```python
from build123d import *

# Parameters (mm, degrees)
SKETCH_1_W          = 200
SKETCH_1_H          = 180
EXTRUDE_1_DEPTH     = 3
SKETCH_2_R          = 1.5
CUT_EXTRUDE_1_DEPTH = 3
SKETCH_3_R          = 1.5
CUT_EXTRUDE_2_DEPTH = 3
SKETCH_4_R          = 2.137012609
SKETCH_4_R_2        = 2.00688496
SKETCH_4_R_3        = 1.920113274
CUT_EXTRUDE_3_DEPTH = 3


with BuildPart() as part:
    # 草图1 → 凸台-拉伸1 (new body)
    with BuildSketch(Plane(origin=(0, 0, 0), x_dir=(1, 0, 0), z_dir=(0, 1, 0))):
        Rectangle(SKETCH_1_W, SKETCH_1_H)
    extrude(amount=EXTRUDE_1_DEPTH)

    # 草图2 → 切除-拉伸1 (cut)
    with BuildSketch(Plane(origin=(0, 3, 0), x_dir=(1, 0, 0), z_dir=(0, 1, 0))):
        with Locations(Location((91.756220162, 76.163438047, 0), (0, 0, 270))):
            Circle(SKETCH_2_R)
        with Locations(Location((91.756220162, 11.939610887, 0), (0, 0, 270))):
            Circle(SKETCH_2_R)
        with Locations(Location((91.756220162, -50.625190386, 0), (0, 0, 270))):
            Circle(SKETCH_2_R)
        with Locations(Location((-91.756220162, 76.163438047, 0), (0, 0, 90))):
            Circle(SKETCH_2_R)
        with Locations(Location((-91.756220162, 11.939610887, 0), (0, 0, 90))):
            Circle(SKETCH_2_R)
        with Locations(Location((-91.756220162, -50.625190386, 0), (0, 0, 90))):
            Circle(SKETCH_2_R)
    extrude(amount=-CUT_EXTRUDE_1_DEPTH, mode=Mode.SUBTRACT)

    # 草图3 → 切除-拉伸2 (cut)
    with BuildSketch(Plane(origin=(0, 3, 0), x_dir=(1, 0, 0), z_dir=(0, 1, 0))):
        with Locations(Location((14.144450177, -3.083468073, 0), (0, 0, 270))):
            Circle(SKETCH_3_R)
        with Locations(Location((14.144450177, -52.083468073, 0), (0, 0, 270))):
            Circle(SKETCH_3_R)
        with Locations(Location((-43.855549823, -52.083468073, 0), (0, 0, 270))):
            Circle(SKETCH_3_R)
        with Locations(Location((-43.855549823, -3.083468073, 0), (0, 0, 270))):
            Circle(SKETCH_3_R)
    extrude(amount=-CUT_EXTRUDE_2_DEPTH, mode=Mode.SUBTRACT)

    # 草图4 → 切除-拉伸3 (cut)
    with BuildSketch(Plane(origin=(0, 3, 0), x_dir=(1, 0, 0), z_dir=(0, 1, 0))):
        with Locations(Location((48.794365555, 16.180217446, 0), (0, 0, 270))):
            Circle(SKETCH_4_R)
        with Locations(Location((48.28042953, 75.551923117, 0), (0, 0, 270))):
            Circle(SKETCH_4_R_2)
        with Locations(Location((28.035307004, 75.551923117, 0), (0, 0, 270))):
            Circle(SKETCH_4_R_2)
        with Locations(Location((15.78042953, 75.551923117, 0), (0, 0, 270))):
            Circle(SKETCH_4_R_3)
        with Locations(Location((-45.929479507, 75.551923117, 0), (0, 0, 270))):
            Circle(SKETCH_4_R)
        with Locations(Location((-45.929479507, 16.180217446, 0), (0, 0, 270))):
            Circle(SKETCH_4_R)
    extrude(amount=-CUT_EXTRUDE_3_DEPTH, mode=Mode.SUBTRACT)


solid = part.part
```
Geometry: final body of the model. Coordinates: model frame, mm. Coordinates: 2 decimals unless noted, no trailing zeros. Write each question's results on one line, items separated by ' | '. Start each with the question number.
1) Mould query, pull axis Z, two halves, no side actions, for faces 1 (the cylindrical face through (47.494, 1.521, -17.876)), 2 (the flat face through (-1, 3, -1)). Classes: released by +Z, released by -Z, zero draft, split by the parting line, or undercut.
2) First-contact query: pin 1 (1.8 mm diameter, centred on x = 14.14, z = 52.08, fed in from -Y). Flat tip, straight axial feed; report the tip coordinate or a pass-through.
3) Material intervals for line 1 along X through (y, z) = (1.4, 3); line 2 along X through (y, z) = (0.1, -17.5), sorted ascending.
Checks:
1) face 1: undercut | face 2: zero draft
2) pin 1: through
3) line 1: -100 to -45.35, -42.36 to 12.65, 15.64 to 100 | line 2: -100 to -47.61, -44.25 to 47.11, 50.48 to 100
